from build123d import *

# Parameters (mm, degrees)
BOSS_EXTRUDE1_DEPTH      = 2
BOSS_EXTRUDE2_DEPTH      = 13
BOSS_EXTRUDE3_START      = -2
BOSS_EXTRUDE3_DEPTH      = 2
SKETCH4_R                = 12.5
CUT_EXTRUDE2_DEPTH       = 1
SKETCH5_W                = 10
SKETCH5_H                = 3.5
USB_C_CUT_DEPTH          = 4
SKETCH6_R                = 3.5
VOLUME_BUTTONS_CUT_DEPTH = 4


with BuildPart() as part:
    # Sketch1 → Boss-Extrude1 (new body)
    with BuildSketch(Plane(origin=(0, 0, 0), x_dir=(1, 0, 0), z_dir=(0, 1, 0))):
        with BuildLine():
            Line((-25.980762114, 15), (-25.980762114, 30))
            Line((-25.980762114, 30), (0, 30))
            ThreePointArc((0, 30), (15, -25.980762114), (-25.980762114, 15))
        make_face()
    extrude(amount=BOSS_EXTRUDE1_DEPTH)

    # Sketch2 → Boss-Extrude2 (add)
    with BuildSketch(Plane(origin=(0, 2, 0), x_dir=(1, 0, 0), z_dir=(0, 1, 0))):
        with BuildLine():
            Line((0, 30), (-25.980762114, 30))
            Line((-25.980762114, 30), (-25.980762114, 15))
            ThreePointArc((-25.980762114, 15), (15, -25.980762114), (0, 30))
        make_face()
        with BuildLine():
            Line((0, 28), (-23.980762114, 28))
            Line((-23.980762114, 28), (-23.980762114, 14.454170625))
            ThreePointArc((-23.980762114, 14.454170625), (13.77104249, -24.379466539), (0, 28))
        make_face(mode=Mode.SUBTRACT)
    extrude(amount=BOSS_EXTRUDE2_DEPTH)

    # Sketch3 → Boss-Extrude3 (add)
    with BuildSketch(Plane(origin=(0, 15, 0), x_dir=(1, 0, 0), z_dir=(0, 1, 0)).offset(BOSS_EXTRUDE3_START)):
        with BuildLine():
            Line((-23.980762114, 14.454170625), (-23.980762114, 28))
            Line((-23.980762114, 28), (0, 28))
            ThreePointArc((0, 28), (-13.77104249, 24.379466539), (-23.980762114, 14.454170625))
        make_face()
    extrude(amount=BOSS_EXTRUDE3_DEPTH)

    # Sketch4 → Cut-Extrude2 (cut)
    with BuildSketch(Plane.XZ):
        with Locations(Location((0, 0, 0), (0, 0, 270))):
            Circle(SKETCH4_R)
    extrude(amount=-CUT_EXTRUDE2_DEPTH, mode=Mode.SUBTRACT)

    # Sketch5 → USB_C_Cut (cut)
    with BuildSketch(Plane.XY.offset(30)):
        with Locations((0, 7.5)):
            Rectangle(SKETCH5_W, SKETCH5_H)
    extrude(amount=-USB_C_CUT_DEPTH, mode=Mode.SUBTRACT)

    # Sketch6 → Volume_Buttons_Cut (cut)
    with BuildSketch(Plane(origin=(19.283628291, 0, -22.981333294), x_dir=(0, -1, 0), z_dir=(0.642787609686543, 0, -0.7660444431189749))):
        with Locations(Location((-7.5, 4.5, 0), (0, 0, 90))):
            Circle(SKETCH6_R)
        with Locations(Location((-7.5, -4.5, 0), (0, 0, 90))):
            Circle(SKETCH6_R)
    extrude(amount=-VOLUME_BUTTONS_CUT_DEPTH, mode=Mode.SUBTRACT)


solid = part.part
Geometry: final body of the model. Coordinates: model frame, mm. A direction names the side the tool comes from. Coordinates: 2 decimals unless noted, no trailing zeros. Loops run counter-clockwise (first coordinate to the right, second up) from the corner with the lowest first, then second, coordinate; pieces in that order, holes last. Notation, with made-up numbers: M 80,42.5 L 101,42.5 A8 cw 101,53.5 Z; hole C 19.25,83.5 d5. An arc over 180 degrees is marked long. One line per item, written item: value. Start each with the question number.
1) Cut plane B-B (x = -2.5). Return loops of the section in (y, z), then the cut area to 3 significant figures.
2) Pin query (flat end, axial travel): P1, Ø8, axis at x = -10, y = 4, coming from the +Z side; P2, Ø1.6, axis at y = 1, z = -23, coming from the -X side; P3, Ø5, axis at y = 10.5, z = 8.5, coming from the -X side. Return the tip coordinate at first contact, or that it passes through.
3) Draft query along X for faces 6 (the flat face through (0, 1, 0)), 7 (the flat face through (0, 2, 0)), 8 (the flat face through (-13, 7, -30)). Return one class per face: released by +X, released by -X, zero draft, split by the parting line, or undercut.
4) Material intervals for L1, parallel to X at y = 9.25, z = 0; L2, parallel to X at y = 0.35, z = 0, sorted ascending. Write a range as from..to.
5) Reachability of faces 1 (the cylindrical face through (3.755, 0.493, -11.923)), 2 (the flat face through (-13, 0, 0)), 3 (the flat face through (0, 5.75, 29)), 4 (the flat face through (-18, 13, -24)), 5 (the flat face through (-20, 15, -20)) from +Z, -Z, +X, -X, +Y, -Y: full face, straight path, thin tool, end or side. Return the list, or none.
6) Cut plane C-C (x = -15.5). Return loops of the section in (y, z).
7) Cut plane A-A (z = 0). Return loops of the section in (x, y), then the cut area to 3 significant figures.
8) Cut plane D-D (z = 22). Return loops of the section in (x, y), then the cut area to 3 significant figures.
Evaluation:
1. outline: M 0,-30 L 15,-30 L 15,-27.89 L 13,-27.89 L 13,-28 L 2,-28 L 2,27.89 L 5.75,27.89 L 5.75,29.9 L 0,29.9 L 0,12.25 L 1,12.25 L 1,-12.25 L 0,-12.25 Z; M 9.25,27.89 L 15,27.89 L 15,29.9 L 9.25,29.9 Z
1. area: 141 mm^2
2. P1: z = 29.39
2. P2: x = -25.98
2. P3: x = -29.39
3. face 6: undercut
3. face 7: undercut
3. face 8: zero draft
4. L1: -30..-28, 28..30
4. L2: -30..-12.5, 12.5..30
5. face 1: -Y
5. face 2: +Z, -Z, +X, -X, -Y
5. face 3: +Z
5. face 4: none
5. face 5: +Z, -Z, +X, -X, +Y
6. outline: M 0,-30 L 15,-30 L 15,-23.32 L 13,-23.32 L 13,-28 L 2,-28 L 2,23.32 L 15,23.32 L 15,25.69 L 0,25.69 Z
7. outline: M -30,0 L -12.5,0 L -12.5,1 L 12.5,1 L 12.5,0 L 30,0 L 30,15 L 28,15 L 28,2 L -28,2 L -28,15 L -30,15 Z
7. area: 147 mm^2
8. outline: M -20.4,0 L 20.4,0 L 20.4,15 L 17.32,15 L 17.32,2 L -17.32,2 L -17.32,15 L -20.4,15 Z
8. area: 162 mm^2
